Source: three-view drawing plus pictorial views. Frame: mm from the lowest corner of the part. A direction names the side the tool comes from. Round coordinates to 2 decimals unless told otherwise and drop trailing zeros. Write each loop counter-clockwise with the first axis right and the second up, starting at its lowest first coordinate (ties: lowest second). Pieces come first, ordered by that corner, then holes. Notation, with made-up numbers: (52.25, 41.5) - (61.25, 41.5) arc R17 cw to (61.25, 64.5) - close; hole circle Ø2 at (57, 34.5). An arc over 180 degrees is marked (long way). Write each question's results on one line, items separated by ' | '.
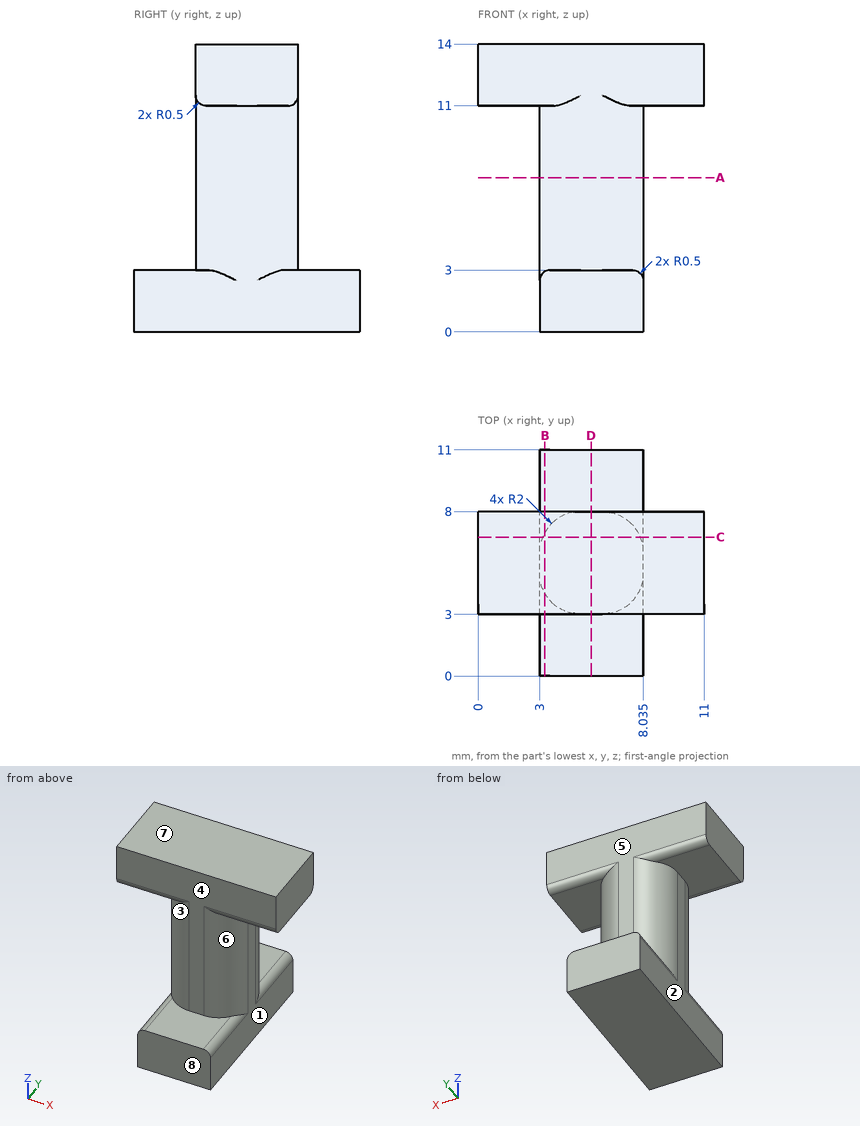
Q1. Ray query, line 1 along X through (y, z) = (5.5, 7.75) (3 decimals); line 2 along Y through (x, z) = (5.25, 6); line 3 along Z through (x, y) = (6.25, 10.5). Return the intervals inside material, ascending.
Answer block:
line 1: 3 to 8.035 | line 2: 3 to 8 | line 3: 0 to 3
Q2. Section query D-D, the plane x = 5.5. Return loops of the section in (y, z).
Answer block:
outline: (0, 0) - (11, 0) - (11, 3) - (8, 3) - (8, 14) - (3, 14) - (3, 3) - (0, 3) - close
Q3. Pin query (flat end, axial travel): pin 1 (3 mm diameter, centred on x = 1, y = 5, fed in from -Z); pin 2 (1.1 mm diameter, centred on x = 5.5, y = 9.5, fed in from +Z); pin 3 (1.1 mm diameter, centred on x = 5, y = 2.5, fed in from +Z); pin 4 (3 mm diameter, centred on x = 8.5, z = 9, fed in from +Y). Return the tip coordinate at first contact, or that it passes through.
Answer block:
pin 1: z = 11 | pin 2: z = 3 | pin 3: z = 14 | pin 4: y = 7.75
Q4. Section query A-A, the plane z = 7.5. Return loops of the section in (x, y) (3 decimals), plus the area to 3 significant figures.
Answer block:
outline: (3, 5) arc R2 ccw to (5, 3) - (6.035, 3) arc R2 ccw to (8.035, 5) - (8.035, 6) arc R2 ccw to (6.035, 8) - (5, 8) arc R2 ccw to (3, 6) - close | area: 21.7 mm2
Q5. Access query for the marked faces 1, 2, 3, 4 and 5. Directions: +Z, -Z, +X, -X, +Y, -Y. A direction counts if a zero-diameter tool reaches every point of the face in a straight line with its end or side. Return the directions, or none.
Answer block:
face 1: -Z, +X, +Y, -Y | face 2: -Z, -X, +Y, -Y | face 3: -X, -Y | face 4: +Z, +X, -X, -Y | face 5: +Z, +X, -X, +Y
Q6. Mould query, pull axis Z, two halves, no side actions, for the marked faces 6, 7 and 8. Classes: pulls with the +Z half, pulls with the -Z half, needs draft (parallel to the pull), parting line crosses it, or undercut.
Answer block:
face 6: undercut | face 7: pulls with the +Z half | face 8: needs draft
Q7. Section query B-B, the plane x = 3.25. Return loops of the section in (y, z).
Answer block:
outline: (0, 0) - (11, 0) - (11, 2.93) - (6.97, 2.93) - (6.97, 11) - (7.5, 11) arc R0.5 ccw to (8, 11.5) - (8, 14) - (3, 14) - (3, 11.5) arc R0.5 ccw to (3.5, 11) - (4.03, 11) - (4.03, 2.93) - (0, 2.93) - close
Q8. Section query C-C, the plane y = 6.75. Return loops of the section in (x, z) (3 decimals).
Answer block:
outline: (0, 11) - (3.146, 11) - (3.146, 2.853) arc R0.5 ccw to (3, 2.5) - (3, 0) - (8.035, 0) - (8.035, 2.5) arc R0.5 ccw to (7.889, 2.853) - (7.889, 11) - (11, 11) - (11, 14) - (0, 14) - close
